Verification items for the finished model (mm, model axes). A direction names the side the tool comes from. Coordinates: 2 decimals unless noted, no trailing zeros. Write each loop counter-clockwise with the first axis right and the second up, starting at its lowest first coordinate (ties: lowest second). Pieces come first, ordered by that corner, then holes. Notation, with made-up numbers: M -24,89.25 L 28,89.25 A15 cw 28,117.25 Z; hole C 45.25,0.25 d5. An arc over 180 degrees is marked long. Answer in a Markdown table with one row per item.
Autodesk Inventor part; units mm, degrees
ref_plane "YZ Plane" through (0, 0, 0) normal (1, 0, 0) x (0, 1, 0)
ref_plane "XZ Plane" through (0, 0, 0) normal (0, 1, 0) x (-1, 0, 0)
ref_plane "XY Plane" through (0, 0, 0) normal (0, 0, 1) x (1, 0, 0)
sketch "Sketch1" plane through (0, 0, 0) normal (0, 1, 0) x (-1, 0, 0)
  line L0 (-28, 28) -> (28, 28)
  line L1 (28, 28) -> (28, -28)
  line L2 (28, -28) -> (-28, -28)
  line L3 (-28, -28) -> (-28, 28)
  line L4 (-28, 28) -> (28, -28) construction
  line L5 (28, 28) -> (-28, -28) construction
  point P0 (0, 0)
  dimension "d0" = 56
  dimension "d1" = 56
extrude "Extrusion1" add sketch "Sketch1" along normal blind 1.6
sketch "Sketch2" plane through (0, 1.6, 0) normal (0, 1, 0) x (1, 0, 0)
  line L0 (25, -25) -> (-25, 25) construction
  line L1 (-25, -25) -> (25, 25) construction
  line L2 (-25, -25) -> (-25, -15)
  line L3 (-25, -15) -> (-24, -15)
  line L4 (-24, -15) -> (-24, -24)
  line L5 (-24, -24) -> (-15, -24)
  line L6 (-15, -24) -> (-15, -25)
  line L7 (15, -24) -> (15, -25)
  line L8 (-25, -25) -> (-15, -25)
  line L9 (-5, -25) -> (-5, -24)
  line L10 (-28, -28) -> (28, -28)
  line L11 (-25, 15) -> (-24, 15)
  line L12 (-25, -5) -> (-24, -5)
  line L13 (-24, -5) -> (-24, 5)
  line L14 (-24, 5) -> (-25, 5)
  line L15 (-25, -5) -> (-25, 5)
  line L16 (-28, 28) -> (-28, -28)
  line L17 (-5, 25) -> (-5, 24)
  line L18 (-5, 24) -> (5, 24)
  line L19 (5, 24) -> (5, 25)
  line L20 (25, 25) -> (15, 25)
  line L21 (15, 25) -> (15, 24)
  line L22 (15, 24) -> (24, 24)
  line L23 (24, 24) -> (24, 15)
  line L24 (24, 15) -> (25, 15)
  line L25 (-5, 25) -> (5, 25)
  line L26 (25, -5) -> (24, -5)
  line L27 (24, -5) -> (24, 5)
  line L28 (24, 5) -> (25, 5)
  line L29 (25, 5) -> (25, -5)
  line L30 (28, 28) -> (-28, 28)
  line L31 (25, 15) -> (25, 25)
  line L32 (15, -25) -> (25, -25)
  line L33 (25, -25) -> (25, -15)
  line L34 (25, -15) -> (24, -15)
  line L35 (24, -15) -> (24, -24)
  line L36 (15, -24) -> (24, -24)
  line L37 (-5, -25) -> (5, -25)
  line L38 (5, -25) -> (5, -24)
  line L39 (5, -24) -> (-5, -24)
  line L40 (-5, -24) -> (-5, -25)
  line L41 (-25, 15) -> (-25, 25)
  line L42 (-25, 25) -> (-15, 25)
  line L43 (-15, 25) -> (-15, 24)
  line L44 (-15, 24) -> (-24, 24)
  line L45 (-24, 15) -> (-24, 24)
  point P0 (0, 0)
  dimension "d4" = 50
  dimension "d5" = 50
  dimension "d6" = 10
  dimension "d7" = 1
  dimension "d8" = 9
  dimension "d9" = 9
  dimension "d16" = 10
  dimension "d17" = 10
  dimension "d18" = 1
  dimension "d21" = 1
  dimension "d22" = 10
  dimension "d23" = 3
  dimension "d24" = 10
  dimension "d25" = 1
  dimension "d27" = 10
  dimension "d28" = 10
  dimension "d29" = 1
  dimension "d30" = 9
  dimension "d31" = 9
  dimension "d32" = 1
  dimension "d33" = 10
  dimension "d34" = 1
  dimension "d35" = 10
  dimension "d36" = 3
  dimension "d37" = 10
  dimension "d38" = 10
  dimension "d39" = 10
  dimension "d40" = 10
  dimension "d41" = 10
extrude "Extrusion2" cut sketch "Sketch2" against normal blind 1.6
sketch "Sketch3" plane through (0, 1.6, 0) normal (0, 1, 0) x (1, 0, 0)
  circle A0 centre (-18.2, 21.5) radius 0.5
  circle A1 centre (21.5, 18.2) radius 0.5
  circle A2 centre (18.2, -21.5) radius 0.5
  circle A3 centre (-21.5, -18.2) radius 0.5
  line L0 (-25, -25) -> (-25, -15)
  line L1 (-15, -25) -> (-25, -25)
  line L2 (-25, 25) -> (-15, 25)
  line L3 (-25, 15) -> (-25, 25)
  line L4 (25, 25) -> (25, 15)
  line L5 (15, 25) -> (25, 25)
  line L6 (25, -15) -> (25, -25)
  line L7 (25, -25) -> (15, -25)
  point P0 (0, 0)
  dimension "d44" = 1
  dimension "d45" = 1
  dimension "d46" = 1
  dimension "d47" = 1
  dimension "d48" = 3.5
  dimension "d49" = 6.8
  dimension "d50" = 3.5
  dimension "d51" = 6.8
  dimension "d52" = 3.5
  dimension "d53" = 6.8
  dimension "d54" = 6.8
  dimension "d55" = 3.5
extrude "Extrusion3" cut sketch "Sketch3" against normal blind 1.6
properties part number "Bottom Panel"
1) Sectioned sample at B-B (x = 0). Record the cut outline in (y, z), then the cut area to 3 significant figures.
Response values:
| item | result |
|---|---|
| outline | M 0,-28 L 1.6,-28 L 1.6,-25 L 0,-25 Z; M 0,-24 L 1.6,-24 L 1.6,24 L 0,24 Z; M 0,25 L 1.6,25 L 1.6,28 L 0,28 Z |
| area | 86.4 mm² |
2) Sectioned sample at A-A (z = -2.5). Record the cut outline in (x, y).
Response values:
| item | result |
|---|---|
| outline | M -28,0 L -25,0 L -25,1.6 L -28,1.6 Z; M -24,0 L 24,0 L 24,1.6 L -24,1.6 Z; M 25,0 L 28,0 L 28,1.6 L 25,1.6 Z |
3) Release check for a two-part mould opening along Z. For faces 3 (the face through (0, 1.6, 0)), 4 (the face through (0, 1, 24)), 5 (the face through (0, 1, -28)) record: +Z half, -Z half, draft (parallel to the pull), parting line (faces both ways), or undercut.
Response values:
| item | result |
|---|---|
| face 3 | draft |
| face 4 | undercut |
| face 5 | -Z half |
4) Tool access check on faces 1 (the face through (-20, 1, 24)), 2 (the face through (28, 1, 0)). Record the directions out of +Z, -Z, +X, -X, +Y, -Y that give a thin tool (end or side, any length) a straight path to the whole face; none if there is none.
Response values:
| item | result |
|---|---|
| face 1 | +Y, -Y |
| face 2 | +Z, -Z, +X, +Y, -Y |
5) Thickness scan on L1, parallel to X at y = 0.85, z = -18.2; L2, parallel to Z at x = -16.5, y = 1.3. Record the ranges inside material, lowest first. Write a range as [from, to].
Response values:
| item | result |
|---|---|
| L1 | x = [-28, -25], [-24, 21], [22, 24], [25, 28] |
| L2 | z = [-28, -25], [-24, 24], [25, 28] |
6) Sectioned sample at C-C (y = 0.75). Give the number of separate pieces and of enclosed holes in the cut face, then the cut area to 3 significant figures.
Response values:
| item | result |
|---|---|
| separate pieces | 1 |
| enclosed holes | 12 |
| area | 3,020 mm² |
